from build123d import *

# Parameters (mm, degrees)
BOSS_EXTRUDE1_DEPTH  = 1.5
SKETCH1_8_R          = 4.1
BOSS_EXTRUDE3_DEPTH  = 36
SKETCH1_9_R          = 5.05
BOSS_EXTRUDE4_DEPTH  = 19
SHELL1_START         = 2
SHELL1_OUTLINE_R     = 2.1
SHELL1_DEPTH         = 32
SHELL1_2_OUTLINE_R   = 3.05
SHELL1_2_OUTLINE_R_2 = 2.1
SHELL1_2_DEPTH       = 15
SKETCH1_10_R         = 3.25
CUT_EXTRUDE1_DEPTH   = 17
SKETCH1_3_R          = 3.25
BOSS_EXTRUDE2_DEPTH  = 6
CHAMFER1_SIZE        = 2
CHAMFER1_SIZE2       = 0.727940469
CHAMFER2_SIZE        = 2.747477419
CHAMFER2_SIZE_2      = 1
CHAMFER3_SIZE        = 1.212435565
CHAMFER3_SIZE_2      = 0.7
CHAMFER6_SIZE        = 0.3
FILLET1_R            = 3.2
CHAMFER5_SIZE        = 0.3
FILLET2_R            = 1
FILLET3_R            = 2


# Read off the part's stored shape, not the designer's step: Shell1
with BuildPart() as part:
    # Sketch1 → Boss-Extrude1 (new body)
    with BuildSketch(Plane.XY):
        Polygon((-10.9, 6.293117934), (0, 12.586235868), (10.9, 6.293117934), (10.9, -6.293117934), (0, -12.586235868), (-10.9, -6.293117934), align=None)
    extrude(amount=BOSS_EXTRUDE1_DEPTH)

    # Sketch1<8> → Boss-Extrude3 (add)
    with BuildSketch(Plane.XY):
        with Locations(Location((0, 0, 0), (0, 0, 180))):
            Circle(SKETCH1_8_R)
    extrude(amount=BOSS_EXTRUDE3_DEPTH)

    # Sketch1<9> → Boss-Extrude4 (add)
    with BuildSketch(Plane.XY):
        with Locations(Location((0, 0, 0), (0, 0, 180))):
            Circle(SKETCH1_9_R)
    extrude(amount=BOSS_EXTRUDE4_DEPTH)

    # Shell1 outline → Shell1 (cut)
    with BuildSketch(Plane.XY.offset(SHELL1_START)):
        Circle(SHELL1_OUTLINE_R)
    extrude(amount=SHELL1_DEPTH, mode=Mode.SUBTRACT)

    # Shell1 2 outline → Shell1 2 (cut)
    with BuildSketch(Plane.XY.offset(SHELL1_START)):
        Circle(SHELL1_2_OUTLINE_R)
        Circle(SHELL1_2_OUTLINE_R_2, mode=Mode.SUBTRACT)
    extrude(amount=SHELL1_2_DEPTH, mode=Mode.SUBTRACT)

    # Sketch1<10> → Cut-Extrude1 (cut)
    with BuildSketch(Plane.XY):
        Circle(SKETCH1_10_R)
    extrude(amount=CUT_EXTRUDE1_DEPTH, mode=Mode.SUBTRACT)

    # Sketch1<3> → Boss-Extrude2 (add)
    with BuildSketch(Plane.XY):
        Polygon((0, 11.547005384), (10, 5.773502692), (10, -5.773502692), (0, -11.547005384), (-10, -5.773502692), (-10, 5.773502692), align=None)
        Circle(SKETCH1_3_R, mode=Mode.SUBTRACT)
    extrude(amount=BOSS_EXTRUDE2_DEPTH)

    # Chamfer1
    chamfer1_edges = [part.edges().sort_by_distance(p)[0] for p in [
        (4.1, 0, 36),
    ]]
    chamfer1_side = [part.faces().sort_by_distance(p)[0] for p in [
        (4.1, 0, 27.5),
    ]]
    chamfer(chamfer1_edges, length=CHAMFER1_SIZE, length2=CHAMFER1_SIZE2, reference=chamfer1_side[0])

    # Chamfer2
    # the kernel refuses this chamfer: 2.747477419, 1 mm, written as the material it adds along each edge
    with BuildSketch(Plane(origin=(0, 0, 19), x_dir=(-1, 0, 0), z_dir=(0, -1, 0))) as chamfer2_piece_1_section:
        Polygon((4.1, -CHAMFER2_SIZE), (4.1 + CHAMFER2_SIZE_2, 0), (4.1, 0), align=None)
    chamfer2_piece_1 = revolve(axis=Axis((0, 0, 19), (0, 0, -1)), mode=Mode.PRIVATE)
    chamfer2_piece_1 = chamfer2_piece_1 & Plane(origin=(0, 0, 20.481947897), x_dir=(-1, 0, 0), z_dir=(0, 0, -1)) * Cylinder(5.05, 21, mode=Mode.PRIVATE)
    add(chamfer2_piece_1)

    # Chamfer3
    # the kernel refuses this chamfer: 1.212435565, 0.7 mm, written as the material it takes off along each edge
    with BuildSketch(Plane(origin=(0, 0, 17), x_dir=(1, 0, 0), z_dir=(0, -1, 0))) as chamfer3_piece_1_section:
        Polygon((2.1 + CHAMFER3_SIZE, 0), (2.1, CHAMFER3_SIZE_2), (2.1, 0), align=None)
    chamfer3_piece_1 = revolve(axis=Axis((0, 0, 17), (0, 0, 1)), mode=Mode.PRIVATE)
    chamfer3_piece_1 = chamfer3_piece_1 & Plane(origin=(0, 0, 17.363214185), x_dir=(1, 0, 0), z_dir=(0, 0, -1)) * Cylinder(3.25, 14, mode=Mode.PRIVATE)
    add(chamfer3_piece_1, mode=Mode.SUBTRACT)

    # Chamfer6
    chamfer6_edges = [part.edges().sort_by_distance(p)[0] for p in [
        (-3.25, 0, 0),
    ]]
    chamfer(chamfer6_edges, length=CHAMFER6_SIZE)

    # Fillet1
    fillet1_edges = [part.edges().sort_by_distance(p)[0] for p in [
        (-10, -5.773502692, 3.75),
        (0, -11.547005384, 3.75),
        (10, -5.773502692, 3.75),
        (10, 5.773502692, 3.75),
        (0, 11.547005384, 3.75),
        (-10, 5.773502692, 3.75),
    ]]
    fillet(fillet1_edges, radius=FILLET1_R)

    # Chamfer5
    chamfer5_edges = [part.edges().sort_by_distance(p)[0] for p in [
        (-5, -8.660254038, 6),
        (5, 8.660254038, 6),
        (-5, 8.660254038, 6),
        (-10, 0, 6),
        (9.571281292, 5.52598183, 6),
        (0, 11.051963661, 6),
        (-9.571281292, 5.52598183, 6),
        (-9.571281292, -5.52598183, 6),
        (0, -11.051963661, 6),
        (9.571281292, -5.52598183, 6),
        (5.45, 9.439676901, 1.5),
        (10.9, 0, 1.5),
        (5.45, -9.439676901, 1.5),
        (-5.45, -9.439676901, 1.5),
        (-10.9, 0, 1.5),
        (-5.45, 9.439676901, 1.5),
        (10, 0, 6),
        (5, -8.660254038, 6),
    ]]
    chamfer(chamfer5_edges, length=CHAMFER5_SIZE)

    # Fillet2
    fillet2_edges = [part.edges().sort_by_distance(p)[0] for p in [
        (10.9, 6.293117934, 0.6),
        (10.9, -6.293117934, 0.6),
        (0, -12.586235868, 0.6),
        (-10.9, -6.293117934, 0.6),
        (-10.9, 6.293117934, 0.6),
        (0, 12.586235868, 0.6),
    ]]
    fillet(fillet2_edges, radius=FILLET2_R)

    # Fillet3
    fillet3_edges = [part.edges().sort_by_distance(p)[0] for p in [
        (5.05, 0, 6),
    ]]
    fillet(fillet3_edges, radius=FILLET3_R)


solid = part.part
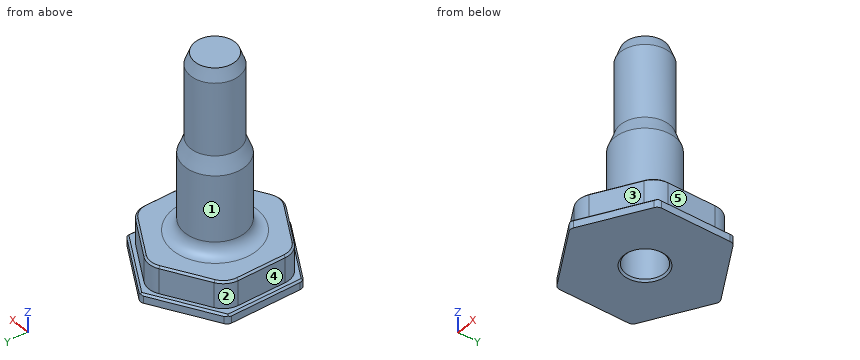
The listing builds one solid part. Answer for the finished solid, in the listing's coordinates (mm). Face numbers are marked on the shaded views. A direction names the side the tool comes from. Coordinates: 2 decimals unless noted, no trailing zeros. Order: outer loops, then holes, each group sorted by start corner. A loop starts at its lowest first (then second) coordinate and runs counter-clockwise, first axis right, second up.
Q1. Which of the six approach directions +Z, -Z, +X, -X, +Y, -Y give full straight-line access (tool end or side, diameter ignored) to the marked faces 1, 2, 3, 4 and 5?
Q2. A cutting plane is placed at C-C, the plane z = 11. Write down the section's boundary in (x, y).
Q3. A cutting plane is placed at A-A, the plane z = 33. Write down the section's boundary in (x, y).
Q4. Consider line 1 (Y direction, x = 0, z = 29.5); line 2 (Y direction, x = 0, z = 17); line 3 (X direction, y = -0.25, z = 16). Determine where each line is inside the solid, lowest interval first.
Q5. Given P1, Ø10, axis at x = -5.5, z = 15, coming from the +Y side; P2, Ø2, axis at y = -1.5, z = 16, coming from the -X side; P3, Ø10, axis at x = 8, z = 22.5, coming from the +Y side, each flat-ended and moving along its own axis, determine where each tip first touches the part or whether it passes through.
Answers follow:
1. face 1: +Z
1. face 2: +Z, -X, +Y
1. face 3: +Z, +X, -Y
1. face 4: +Z, -X, +Y, -Y
1. face 5: +Z, +X, +Y, -Y
2. outline: circle Ø10.1 at (0, 0); hole circle Ø6.5 at (0, 0)
3. outline: circle Ø8.2 at (0, 0); hole circle Ø4.2 at (0, 0)
4. line 1: y = -4.1 to -2.1, 2.1 to 4.1
4. line 2: y = -5.05 to -3.25, 3.25 to 5.05
4. line 3: x = -5.04 to -3.24, 3.24 to 5.04
5. P1: stops at y = 5.03
5. P2: stops at x = -5.03
5. P3: stops at y = 3.01
